from build123d import *

# Parameters (mm, degrees)
SKETCH1_W           = 12
SKETCH1_H           = 4.1
BOSS_EXTRUDE1_DEPTH = 3.7
CUT_EXTRUDE1_DEPTH  = 3.7
CUT_EXTRUDE2_DEPTH  = 3.7
SKETCH5_R           = 1.3
BOSS_EXTRUDE2_DEPTH = 0.4
FILLET1_R           = 0.5
SKETCH6_W           = 10
SKETCH6_H           = 3.1
CUT_EXTRUDE3_DEPTH  = 19.226253597


with BuildPart() as part:
    # Sketch1 → Boss-Extrude1 (new body)
    with BuildSketch(Plane.XY):
        with Locations((-6, 11.160084034)):
            Rectangle(SKETCH1_W, SKETCH1_H)
    extrude(amount=BOSS_EXTRUDE1_DEPTH)

    # Sketch3 → Cut-Extrude1 (cut)
    with BuildSketch(Plane.XY.offset(3.7)):
        Polygon((-1, 13.210084034), (0, 13.210084034), (0, 12.210084034), align=None)
    extrude(amount=-CUT_EXTRUDE1_DEPTH, mode=Mode.SUBTRACT)

    # Sketch4 → Cut-Extrude2 (cut)
    with BuildSketch(Plane.XY.offset(3.7)):
        Polygon((-12, 13.210084034), (-11, 13.210084034), (-12, 12.210084034), align=None)
    extrude(amount=-CUT_EXTRUDE2_DEPTH, mode=Mode.SUBTRACT)

    # Sketch5 → Boss-Extrude2 (add)
    with BuildSketch(Plane.XZ.offset(-9.110084034)):
        with Locations(Location((-6, 1.7, 0), (0, 0, 270))):
            Circle(SKETCH5_R)
    extrude(amount=BOSS_EXTRUDE2_DEPTH)

    # Fillet1
    # the kernel refuses this fillet: 0.5 mm, written as the material it takes off along each edge
    with BuildSketch(Plane(origin=(-6, 8.710084034, 1.7), x_dir=(0, 0, -1), z_dir=(-1, 0, 0))) as fillet1_piece_1:
        with BuildLine():
            CenterArc((0.810102051, -0.5), FILLET1_R, 11.536959033, 78.463040967)
            Line((0.810102051, 0), (0.810102051, 0.01))
            Line((0.810102051, 0.01), (1.3, 0.01))
            Line((1.3, 0.01), (1.31, 0))
            ThreePointArc((1.31, 0), (1.31, -0.2), (1.309797959, -0.398))
            Line((1.309797959, -0.398), (1.3, -0.4))
        make_face()
    revolve(axis=Axis((-6, 8.710084034, 1.7), (0, -1, 0)), mode=Mode.SUBTRACT)

    # Sketch6 → Cut-Extrude3 (cut, through all)
    with BuildSketch(Plane.XY.offset(3.7)):
        with Locations((-6, 11.660084034)):
            Rectangle(SKETCH6_W, SKETCH6_H)
    extrude(amount=-CUT_EXTRUDE3_DEPTH, mode=Mode.SUBTRACT)


solid = part.part
Part model, mm, in its own coordinate system. A direction names the side the tool comes from. Coordinates: 2 decimals unless noted, no trailing zeros. Loops run counter-clockwise (first coordinate to the right, second up) from the corner with the lowest first, then second, coordinate; pieces in that order, holes last. Notation, with made-up numbers: (15, 79) -> (50, 79) arc R29 cw to (50, 103) -> close; hole circle Ø3 at (46, 74). An arc over 180 degrees is marked (long way). Use a Markdown table: item, result. Add a question column.
Item 1: Band-saw the part on B-B on z = 3.4. Write the cut outline in (x, y).
Item 2: Which spindle directions (+Z, -Z, +X, -X, +Y, -Y) get a long thin tool onto all of the face, cutting with end or side? Do faces 1 (the flat face through (-6, 10.11, 2)), 2 (the flat face through (-6.1, 9.8, 3.7)). Say none if no direction does.
Item 3: Band-saw the part on D-D on y = 9. Write the cut outline in (x, z), plus the area to 3 significant figures.
Item 4: Probe probe 1 along X at (y, z) = (10.3, 1.7); probe 2 along Y at (x, z) = (-10.5, 1.35); probe 3 along X at (y, z) = (12.7, 1.2). List the from-to ranges inside material, lowest first.
Item 5: Pull direction X, two halves, no side cores. Call faces 3 (the flat face through (-1, 12, 2)), 4 (the flat face through (-7.4, 9.11, 2.2)), 5 (the flat face through (-12, 11, 2)): +X half, -X half, draft (parallel to the pull), parting line (faces both ways), or undercut.
Item 6: Band-saw the part on A-A on y = 11. Write the cut outline in (x, z), plus the area to 3 significant figures.
Item 7: Flat gauge pin, fed straight in: P1, Ø1, axis at x = -4, z = 1, coming from the +Y side. Where does the tip first touch, or does it go through?
Item 8: Band-saw the part on C-C on x = -10.75. Write the cut outline in (y, z).
Geometry says:
| question | item | result |
|---|---|---|
| 1 | outline | (-12, 9.11) -> (0, 9.11) -> (0, 12.21) -> (-1, 13.21) -> (-1, 10.11) -> (-11, 10.11) -> (-11, 13.21) -> (-12, 12.21) -> close |
| 2 | face 1 | +Z, -Z, +Y |
| 2 | face 2 | +Z, +X, -X, +Y, -Y |
| 3 | outline | circle Ø2.53 at (-6, 1.7) |
| 3 | area | 5.02 mm² |
| 4 | probe 1 | -12 to -11, -1 to 0 |
| 4 | probe 2 | 9.11 to 10.11 |
| 4 | probe 3 | -11.51 to -11, -1 to -0.49 |
| 5 | face 3 | undercut |
| 5 | face 4 | draft |
| 5 | face 5 | -X half |
| 6 | outline | (-12, 0) -> (-11, 0) -> (-11, 3.7) -> (-12, 3.7) -> close; (-1, 0) -> (0, 0) -> (0, 3.7) -> (-1, 3.7) -> close |
| 6 | area | 7.40 mm² |
| 7 | P1 | y = 10.11 |
| 8 | outline | (9.11, 0) -> (10.11, 0) -> (10.11, 3.7) -> (9.11, 3.7) -> close |
